Source: CAD feature listing. Evaluate the final solid. Frame: model axes, mm. Face numbers are marked on the shaded views. Round coordinates to 2 decimals unless told otherwise and drop trailing zeros. Loops run counter-clockwise (first coordinate to the right, second up) from the corner with the lowest first, then second, coordinate; pieces in that order, holes last. Notation, with made-up numbers: M -17.5,-3 L 34.5,-3 A11 cw 34.5,12 Z; hole C -40,45 d4. An arc over 180 degrees is marked long. Write each question's results on one line, items separated by ' | '. Start each with the question number.
1. Section B-B on y = 0. Output: boundary loops of the cut face in (x, z), and give its area (3 significant figures).
2. Ray query, line 1 (Z direction, x = 22.5, y = 0); line 2 (X direction, y = 9.5, z = 6); line 3 (Z direction, x = 17, y = 3). Return the intervals inside material, ascending.
3. Section D-D on x = -15. Output: boundary loops of the cut face in (y, z), and give its area (3 significant figures).
4. Section C-C on z = -4. Output: boundary loops of the cut face in (x, y).
5. Contact query for flat-ended pins moving along their axis: pin 1 Ø2.5 at (y, z) = (0, -4.5) entering from +X; pin 2 Ø1 at (x, y) = (-1.5, -7) entering from +Z; pin 3 Ø6.5 at (x, z) = (-12, -6.5) entering from -Y; pin 4 Ø8 at (x, z) = (-1.5, -20.5) entering from +Y. Output: stop coordinate, or through.
6. Section A-A on y = 9.5. Output: boundary loops of the cut face in (x, z).
7. Draft query along X for the marked faces 1, 2, 3 and 4. Return one class per face: released by +X, released by -X, zero draft, split by the parting line, or undercut.
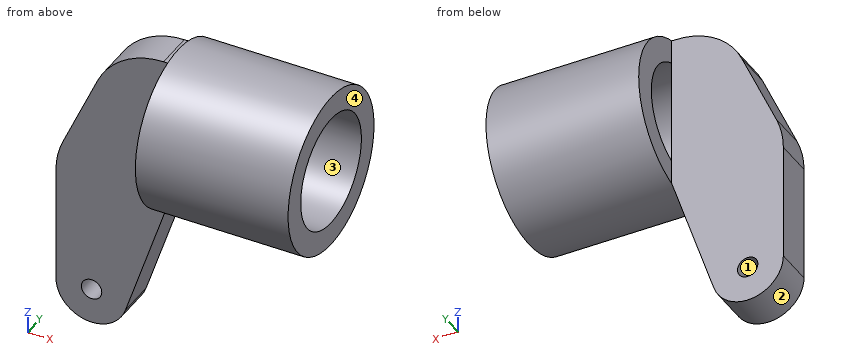
from build123d import *

# Parameters (mm, degrees)
RECTANGLE001_W   = 30
RECTANGLE001_H   = 7.5
EXTRUDE003_DEPTH = 60
SKETCH_R         = 2
EXTRUDE002_DEPTH = 15
SKETCH001_R      = 15.572723
SKETCH001_R_2    = 11
EXTRUDE_DEPTH    = 30


with BuildPart() as extrude003:
    # Rectangle001 → Extrude003 (new body)
    with BuildSketch(Plane(origin=(-30, -3.75, -15), x_dir=(1, 0, 0), z_dir=(0, 0, 1))):
        with Locations((15, 3.75)):
            Rectangle(RECTANGLE001_W, RECTANGLE001_H)
    extrude(amount=EXTRUDE003_DEPTH)


with BuildPart() as extrude003_1:
    # Extrude003 placement: moved
    add(extrude003.part.moved(Location((0, 0, -30))))


with BuildPart() as common:
    # Sketch → Extrude002 (new body)
    with BuildSketch(Plane(origin=(0, 0, -15), x_dir=(1, 0, 0), z_dir=(0, -1, 0))):
        with BuildLine():
            Line((-22, -23), (-22, 0))
            ThreePointArc((-20.644937, 6.353045), (-21.657467, 3.247975), (-22, 0))
            Line((-20.644937, 6.353045), (-13.834191, 21.592376))
            ThreePointArc((-0.867585, 30), (-8.594503, 27.714145), (-13.834191, 21.592376))
            Line((-0.867585, 30), (0, 30))
            Line((0, 30), (0, 0))
            Line((-8.355642, -25.202842), (0, 0))
            ThreePointArc((-22, -23), (-16.115683, -29.910517), (-8.355642, -25.202842))
        make_face()
        with Locations((-15, -23)):
            Circle(SKETCH_R, mode=Mode.SUBTRACT)
    extrude(amount=-EXTRUDE002_DEPTH)


with BuildPart() as common_1:
    # Extrude002 placement: moved
    add(common.part.moved(Location((0, -7.5, 0))))

    # Common: intersect Extrude003
    add(extrude003_1.part, mode=Mode.INTERSECT)


with BuildPart() as body:
    # Sketch001 → Extrude (new body)
    with BuildSketch(Plane.YZ):
        Circle(SKETCH001_R)
        Circle(SKETCH001_R_2, mode=Mode.SUBTRACT)
    extrude(amount=EXTRUDE_DEPTH)

    # Fusion: union Common
    add(common_1.part)


solid = body.part
Taken from the geometry:
1) outline: M -22,-38 A7 ccw -8.36,-40.2 L 0,-15 L 0,-15.57 L 30,-15.57 L 30,-11 L 0,-11 L 0,11 L 30,11 L 30,15.57 L 0,15.57 L 0,15 L -0.87,15 A14.2 ccw -13.83,6.59 L -20.64,-8.65 A15.57 ccw -22,-15 Z; hole C -15,-38 d4 | area: 1,240 mm^2
2) line 1: -15.57 to -11, 11 to 15.57 | line 2: 0 to 30 | line 3: -15.28 to -10.58, 10.58 to 15.28
3) outline: M -3.75,-45 L 3.75,-45 L 3.75,-40 L -3.75,-40 Z; M -3.75,-36 L 3.75,-36 L 3.75,3.98 L -3.75,3.98 Z | area: 337 mm^2
4) outline: M -18.57,-3.75 L 0,-3.75 L 0,3.75 L -18.57,3.75 Z; M 0,-15.05 L 30,-15.05 L 30,-10.25 L 0,-10.25 Z; M 0,10.25 L 30,10.25 L 30,15.05 L 0,15.05 Z
5) pin 1: x = 0 | pin 2: through | pin 3: y = -3.75 | pin 4: y = 3.75
6) outline: M 0,-12.34 L 30,-12.34 L 30,-5.55 L 0,-5.55 Z; M 0,5.55 L 30,5.55 L 30,12.34 L 0,12.34 Z
7) face 1: undercut | face 2: split by the parting line | face 3: zero draft | face 4: released by +X
